from build123d import *

# Parameters (mm, degrees)
EXTRUDE1_DEPTH      = 95.631
EXTRUDE1_DEPTH_BACK = 95.631
SKETCH1_R           = 10.922
SKETCH3_W           = 0.762
SKETCH3_H           = 0.762
RODHOLE_START       = -161.631
SKETCH8_R           = 3.175
RODHOLE_DEPTH       = 161.631
SKETCH9_R           = 9.525
STROKECHAMBER_DEPTH = 106.6
CHAMFER1_SIZE       = 0.5
FLATS_DEPTH         = 110.426622599
FLATS_DEPTH_BACK    = 110.426622599
SKETCH4_W           = 1.397
SKETCH4_H           = 12.7
SKETCH4_W_2         = 0.5
SKETCH4_H_2         = 3.048
ENDFLATS_DEPTH      = 110.426622599
ENDFLATS_DEPTH_BACK = 110.426622599
SKETCH12_W          = 6.096
SKETCH12_H          = 15.024


with BuildPart() as part:
    # Sketch1 → Extrude1 (new, two sides: drawn at the far end of the back side and taken through both)
    with BuildSketch(Plane.XY.offset(-EXTRUDE1_DEPTH_BACK)):
        Circle(SKETCH1_R)
    extrude(amount=EXTRUDE1_DEPTH + EXTRUDE1_DEPTH_BACK)

    # Sketch2 → Nose (revolve)
    with BuildSketch(Plane(origin=(0, 0, 0), x_dir=(0, 0, -1), z_dir=(1, 0, 0)), mode=Mode.PRIVATE) as nose_sk:
        Polygon((-95.631, 7.9248), (-97.917, 7.9248), (-97.917, 7), (-100.717, 7), (-100.717, 7.9375), (-108.331, 7.9375), (-108.331, 0), (-95.631, 0), align=None)
    revolve(nose_sk.sketch.rotate(Axis((0, 0, 0), (0, 0, 1)), 90), axis=Axis((0, 0, 0), (0, 0, 1)))

    # Sketch3 → CoverGrooves (revolve, cut)
    with BuildSketch(Plane(origin=(0, 0, 0), x_dir=(0, 0, -1), z_dir=(1, 0, 0)), mode=Mode.PRIVATE) as covergrooves_sk:
        with Locations((-76.2, 10.541)):
            Rectangle(SKETCH3_W, SKETCH3_H)
        Polygon((-75.057, 10.922), (-75.057, 10.16), (-74.295, 10.16), (-73.533, 10.922), align=None)
        Polygon((65.107, 10.922), (65.107, 10.16), (64.345, 10.922), align=None)
        Polygon((63.583, 10.922), (63.583, 10.16), (62.821, 10.922), align=None)
    revolve(covergrooves_sk.sketch.rotate(Axis((0, 0, 0), (0, 0, 1)), 90), axis=Axis((0, 0, 0), (0, 0, 1)), mode=Mode.SUBTRACT)

    # Sketch7 → FrontPort (revolve, cut)
    with BuildSketch(Plane(origin=(0, 0, 0), x_dir=(0, 0, -1), z_dir=(1, 0, 0))):
        Polygon((-84.201, 10.922), (-78.351, 10.922), (-79.051, 10.222), (-79.051, 0), (-84.201, 0), align=None)
    revolve(axis=Axis((0, 0, 84.201), (0, 1, 0)), mode=Mode.SUBTRACT)

    # Sketch8 → RodHole (cut)
    with BuildSketch(Plane.XY.offset(108.331).offset(RODHOLE_START)):
        Circle(SKETCH8_R)
    extrude(amount=RODHOLE_DEPTH, mode=Mode.SUBTRACT)

    # Sketch9 → StrokeChamber (cut)
    with BuildSketch(Plane.XY.offset(-53.3)):
        Circle(SKETCH9_R)
    extrude(amount=STROKECHAMBER_DEPTH, mode=Mode.SUBTRACT)

    # Chamfer1
    chamfer1_edges = [part.edges().sort_by_distance(p)[0] for p in [
        (-10.922, 0, -95.631),
        (-3.175, 0, 108.331),
        (-10.922, 0, 95.631),
        (7.9375, 0, 108.331),
    ]]
    chamfer(chamfer1_edges, length=CHAMFER1_SIZE)

    # Sketch4 → Flats (cut, two sides: drawn at the far end of the back side and taken through both)
    with BuildSketch(Plane(origin=(0, 0, 0), x_dir=(1, 0, 0), z_dir=(0, 1, 0)).offset(-FLATS_DEPTH_BACK)):
        with Locations((10.2235, -89.281)):
            Rectangle(SKETCH4_W, SKETCH4_H)
        with Locations((10.672, 94.107)):
            Rectangle(SKETCH4_W_2, SKETCH4_H_2)
        with Locations((-10.672, 94.107)):
            Rectangle(SKETCH4_W_2, SKETCH4_H_2)
        with Locations((-10.2235, -89.281)):
            Rectangle(SKETCH4_W, SKETCH4_H)
    extrude(amount=FLATS_DEPTH + FLATS_DEPTH_BACK, mode=Mode.SUBTRACT)

    # Sketch11 → EndThreads (revolve, cut)
    with BuildSketch(Plane(origin=(0, 0, 0), x_dir=(0, 0, -1), z_dir=(1, 0, 0)), mode=Mode.PRIVATE) as endthreads_sk:
        Polygon((95.631, 7.4375), (95.131, 7.9375), (83.07, 7.9375), (83.07, 7), (82.169, 7), (82.169, 7.9375), (79.883, 7.9375), (79.883, 10.16), (79.121, 10.922), (95.631, 10.922), align=None)
    revolve(endthreads_sk.sketch.rotate(Axis((0, 0, 0), (0, 0, -1)), 90), axis=Axis((0, 0, 0), (0, 0, -1)), mode=Mode.SUBTRACT)

    # Sketch13 → RearTopPort (revolve, cut)
    with BuildSketch(Plane(origin=(0, 0, 0), x_dir=(0, 0, -1), z_dir=(1, 0, 0))):
        Polygon((72.771, 0), (77.921, 0), (77.921, 10.222), (78.621, 10.922), (72.771, 10.922), align=None)
    revolve(axis=Axis((0, 0, -72.771), (0, 1, 0)), mode=Mode.SUBTRACT)

    # Sketch12 → EndFlats (cut, two sides: drawn at the far end of the back side and taken through both)
    with BuildSketch(Plane(origin=(0, 0, 0), x_dir=(0, -1, 0), z_dir=(1, 0, 0)).offset(-ENDFLATS_DEPTH_BACK)):
        with Locations((7.874, 88.119)):
            Rectangle(SKETCH12_W, SKETCH12_H)
        with Locations((-7.874, 88.119)):
            Rectangle(SKETCH12_W, SKETCH12_H)
    extrude(amount=ENDFLATS_DEPTH + ENDFLATS_DEPTH_BACK, mode=Mode.SUBTRACT)

    # Sketch15 → ClevisPinHole (revolve, cut)
    with BuildSketch(Plane(origin=(0, 0, 0), x_dir=(0, -1, 0), z_dir=(1, 0, 0)), mode=Mode.PRIVATE) as clevispinhole_sk:
        Polygon((4.826, 92.2067), (4.326, 91.7067), (-4.326, 91.7067), (-4.826, 92.2067), (-4.826, 88.519), (4.826, 88.519), align=None)
    revolve(clevispinhole_sk.sketch.rotate(Axis((0, 0, -88.519), (0, -1, 0)), 180), axis=Axis((0, 0, -88.519), (0, -1, 0)), mode=Mode.SUBTRACT)


solid = part.part
Here's how the part is built. I have some questions about the finished solid (model axes, mm). A direction names the side the tool comes from. Give positions to 0.01 mm unless a question says otherwise; leave off trailing zeros. Loops run counter-clockwise (first coordinate to the right, second up) from the corner with the lowest first, then second, coordinate; pieces in that order, holes last. Notation, with made-up numbers: (-32.75, 70) -> (-27.75, 70) arc R33 cw to (-27.75, 100) -> close; hole circle Ø10 at (77, 84.5). An arc over 180 degrees is marked (long way). One line per item, written item: value.
Q1. I'm going to push flat-ended pins straight in: pin 1 Ø4 at (x, z) = (2, -89.5) entering from +Y; pin 2 Ø10 at (x, y) = (-4.5, 5.5) entering from -Z; pin 3 Ø2 at (x, z) = (-8.5, 20.5) entering from +Y; pin 4 Ø3 at (x, y) = (3.5, -7) entering from -Z. Where does each tip first touch, or does it pass through?
Answers follow:
pin 1: y = 4.83
pin 2: z = -95.63
pin 3: y = 7.94
pin 4: z = -80.61
Q2. Suppose I cut it at B-B on x = 0. State how many separate pieces and enclosed holes the cut face has, then the cut area to 3 significant figures.
Answers follow:
separate pieces: 3
enclosed holes: 0
area: 1,550 mm^2
Q3. Suppose I cut it at A-A on z = -4. Please give me the cut outline in (x, y) (3 decimals), then the cut area to 3 significant figures.
Answers follow:
outline: circle Ø21.844 at (0, 0); hole circle Ø19.05 at (0, 0)
area: 89.7 mm^2
Q4. Suppose I cut it at C-C on z = 62.5. Please give me the cut outline in (x, y) (3 decimals).
Answers follow:
outline: circle Ø21.844 at (0, 0); hole circle Ø6.35 at (0, 0)
Q5. On a 3-axis mill with a long thin cutter (end or side, diameter ignored), from which of +Z, -Z, +X, -X, +Y, -Y can I reach the whole of each face in a straight line? I mean faces 1 (the face through (-0.226, 5.039, 89.346)), 2 (the face through (6.8, 4.5, -79.883)), 3 (the face through (-0.69, -3.1, 80.18)), 4 (the face through (-4, 6, 97.917)). Say none if no direction works.
Answers follow:
face 1: +Y
face 2: -Z
face 3: +Z
face 4: none
Q6. We'd pull the mould along Y, two halves only. Please class faces 5 (the face through (4, 0, 53.3)), 6 (the face through (-0.09, -4.826, -84.68)), 7 (the face through (-7.937, -0.073, -89.016)): pulls with the +Y half, pulls with the -Y half, needs draft (parallel to the pull), parting line crosses it, or undercut.
Answers follow:
face 5: undercut
face 6: pulls with the -Y half
face 7: parting line crosses it
Q7. If I drill on line 1 along Z through (x, y) = (6, -2.75); line 2 along Z through (x, y) = (1.25, 6.75) (3 decimals); line 3 along X through (y, z) = (0, 95.5) (3 decimals), over which ranges is the centre line in solid material (lowest first)?
Answers follow:
line 1: -95.63 to -53.3, 53.3 to 108.33
line 2: -80.607 to -77.767, -67.775 to -53.3, 53.3 to 79.205, 89.197 to 108.331
line 3: -9.525 to -3.175, 3.175 to 9.525
